Part model, mm, in its own coordinate system. A direction names the side the tool comes from. Round coordinates to 2 decimals unless told otherwise and drop trailing zeros. Loops run counter-clockwise (first coordinate to the right, second up) from the corner with the lowest first, then second, coordinate; pieces in that order, holes last.
1) Band-saw the part on B-B, the plane x = -31.75. Write the cut outline in (y, z).
2) Mould opens along X. For faces 3 (the flat face through (0, -1, 9)), 4 (the flat face through (-18, 1, 19.05)), 5 (the cylindrical face through (-35.28, 14.39, 9.39)), 6 (the cylindrical face through (-31.61, -6.35, 9.39)) say: +X half, -X half, draft (parallel to the pull), parting line (faces both ways), or undercut.
3) Probe line 1 (X direction, y = 4, z = 12.5); line 2 (X direction, y = 6, z = 12); line 3 (Y direction, x = -19.5, z = 7.25). List the from-to ranges inside material, lowest first.
4) 3-axis set-ups, long thin cutter, end or side, ignore diameter. For faces 1 (the flat face through (-18, 1, 0)), 2 (the cylindrical face through (-23.413, 9.849, 9.392)): which of +Z, -Z, +X, -X, +Y, -Y reach the whole face in a straight line?
5) Band-saw the part on A-A, the plane z = 17.75. Write the cut outline in (x, y).
6) Band-saw the part on D-D, the plane x = -14. Write the cut outline in (y, z).
7) Drop flat-ended pins along their axis: P1, Ø3, axis at y = 2, z = 5, coming from the -X side; P2, Ø3, axis at x = -8, z = 10.5, coming from the +Y side; P3, Ø1, axis at x = -13.5, y = -34.5, coming from the -Z side; P4, Ø10, axis at x = -8.5, z = 2, coming from the +Y side. Give the stop position or say it passes through.
8) Band-saw the part on C-C, the plane y = 34. Write the cut outline in (x, z), then the cut area to 3 significant figures.
from build123d import *

# Parameters (mm, degrees)
F1_DEPTH = 19.05


with BuildPart() as f1:
    # F0 (on Top) → F1 (new body)
    with BuildSketch(Plane.XY):
        with BuildLine():
            Line((0, 38.1), (0, 44.45))
            ThreePointArc((0, 44.45), (-31.430896, 31.430896), (-44.45, 0))
            ThreePointArc((-44.45, 0), (-31.430896, -31.430896), (0, -44.45))
            Line((0, -44.45), (0, -38.1))
            Line((0, -38.1), (0, -25.4))
            Line((0, -25.4), (0, 25.4))
            Line((0, 25.4), (0, 38.1))
        make_face()
        with BuildLine():
            ThreePointArc((-25.4, 0), (-31.75, -6.35), (-38.1, 0))
            ThreePointArc((-38.1, 0), (-35.19981, 14.580239), (-26.940768, 26.940768))
            ThreePointArc((-26.940768, 26.940768), (-17.960512, 26.940768), (-17.960512, 17.960512))
            ThreePointArc((-17.960512, 17.960512), (-23.46654, 9.720159), (-25.4, 0))
        make_face(mode=Mode.SUBTRACT)
    extrude(amount=F1_DEPTH)


solid = f1.part
Reported:
1. outline: (-31.11, 0) - (-6.35, 0) - (-6.35, 19.05) - (-31.11, 19.05) - close; (21.06, 0) - (31.11, 0) - (31.11, 19.05) - (21.06, 19.05) - close
2. face 3: +X half
2. face 4: draft
2. face 5: undercut
2. face 6: undercut
3. line 1: x = -44.27 to -37.89, -25.08 to 0
3. line 2: x = -44.04 to -37.62, -24.68 to 0
3. line 3: y = -39.94 to 16.28, 28.07 to 39.94
4. face 1: -Z, +X, -X, +Y, -Y
4. face 2: +Z, -Z
5. outline: (-44.45, 0) arc R44.45 ccw to (0, -44.45) - (0, 44.45) arc R44.45 ccw to start; hole (-38.1, 0) arc R6.35 ccw to (-25.4, 0) arc R25.4 cw to (-17.96, 17.96) arc R6.35 ccw to (-26.94, 26.94) arc R38.1 ccw to start
6. outline: (-42.19, 0) - (42.19, 0) - (42.19, 19.05) - (-42.19, 19.05) - close
7. P1: stops at x = -44.45
7. P2: stops at y = 43.97
7. P3: stops at z = 0
7. P4: stops at y = 44.31
8. outline: (-28.63, 0) - (0, 0) - (0, 19.05) - (-28.63, 19.05) - close
8. area: 545 mm2
